Here's how the part is built. I have some questions about the finished solid (model axes, mm). Round coordinates to 2 decimals unless told otherwise and drop trailing zeros. Write each loop counter-clockwise with the first axis right and the second up, starting at its lowest first coordinate (ties: lowest second). Pieces come first, ordered by that corner, then holes. Notation, with made-up numbers: (-24, 23) - (6, 23) arc R26 ccw to (6, 48) - close; hole circle Ø8 at (8.5, 84.25). An arc over 180 degrees is marked (long way). One line per question, with ' | ' between items. Start each with the question number.
(1) Imagine slicing it at A-A (y = 79). Write out the boundary of the cut face in (x, z), plus the area to 3 significant figures.
(2) Thinking about a two-plate mould opening in Z: for faces 1 (the cylindrical face through (10.99, 81.2, -249.76)), 2 (the flat face through (3, 150, -3)), 3 (the flat face through (3, 25, -3)), which applies, pulls with the +Z half, pulls with the -Z half, needs draft (parallel to the pull), parting line crosses it, or undercut?
(3) Will these pins go through, and if not, where does the flat tip stop? pin 1 (12 mm diameter, centred on x = -47, y = 124.5, fed in from +Z); pin 2 (1.5 mm diameter, centred on x = -129.5, y = 117, fed in from -Z); pin 3 (6 mm diameter, centred on x = 148.5, z = 75.5, fed in from -Y).
(4) If I drill on L1, parallel to Y at x = -16, z = 130; L2, parallel to X at y = 20, z = 2; L3, parallel to X at y = 98, z = -17, over which ranges is the centre line in solid material (lowest first)?
(5) Imagine slicing it at B-B (y = 113.5). Write out the boundary of the cut face in (x, z), plus the area to 3 significant figures.
from build123d import *

# Parameters (mm, degrees)
SKETCH_4_R          = 250
EXTRUDE_2_DEPTH     = 150
FILLET_1_R          = 60
FILLET_2_R          = 47
SKETCH_16_R         = 190
CUT_EXTRUDE_1_DEPTH = 25
FILLET_3_R          = 25


with BuildPart() as part:
    # 草图4 → 凸台-拉伸2 (new body)
    with BuildSketch(Plane(origin=(0, 0, 0), x_dir=(1, 0, 0), z_dir=(0, 1, 0))):
        with Locations(Location((0, 0, 0), (0, 0, 270))):
            Circle(SKETCH_4_R)
    extrude(amount=EXTRUDE_2_DEPTH)

    # 圆角1
    fillet_1_edges = [part.edges().sort_by_distance(p)[0] for p in [
        (0, 0, -250),
    ]]
    fillet(fillet_1_edges, radius=FILLET_1_R)

    # 圆角2
    fillet_2_edges = [part.edges().sort_by_distance(p)[0] for p in [
        (0, 150, -250),
    ]]
    fillet(fillet_2_edges, radius=FILLET_2_R)

    # 草图16 → 切除-拉伸1 (cut)
    with BuildSketch(Plane(origin=(0, 0, 0), x_dir=(1, 0, 0), z_dir=(0, 1, 0))):
        with Locations(Location((0, 0, 0), (0, 0, 270))):
            Circle(SKETCH_16_R)
    extrude(amount=CUT_EXTRUDE_1_DEPTH, mode=Mode.SUBTRACT)

    # 圆角3
    # the kernel refuses this fillet: 25 mm, written as the material it takes off along each edge
    with BuildSketch(Plane(origin=(0, 0, 0), x_dir=(0, 0, 1), z_dir=(-1, 0, 0))) as fillet_3_piece_1:
        with BuildLine():
            CenterArc((213.35124434, 33.928571429), FILLET_3_R, 200.924832428, 110.924832428)
            Line((190, 25), (189.532975113, 24.821428571))
            ThreePointArc((189.532975113, 24.821428571), (189.5, 12.5), (189.5, 0))
            Line((189.5, 0), (190, -0.5))
            ThreePointArc((190, -0.5), (211.607142857, 3.489988696), (230.364293788, 14.933673469))
            Line((230.364293788, 14.933673469), (230.030704584, 15.306122449))
        make_face()
    revolve(axis=Axis((0, 0, 0), (0, 1, 0)), mode=Mode.SUBTRACT)

    # 倒角1
    # the kernel refuses this chamfer: 17.333818879, 10 mm, written as the material it adds along each edge
    with BuildSketch(Plane(origin=(0, 25, 0), x_dir=(0, 0, 1), z_dir=(-1, 0, 0))) as chamfer_1_piece_1:
        with BuildLine():
            Line((197.061199814, -10.000793021), (184.322097601, 0.439495442))
            Line((184.322097601, 0.439495442), (184.322097601, 0.786171819))
            ThreePointArc((184.322097601, 0.786171819), (187.161048801, 0.346676378), (190, 0.346676378))
            Line((190, 0.346676378), (190.323812992, 0.123812992))
            ThreePointArc((190.323812992, 0.123812992), (193.180553266, -5.246391965), (197.294531196, -9.744392989))
            Line((197.294531196, -9.744392989), (197.061199814, -10.000793021))
        make_face()
    revolve(axis=Axis((0, 25, 0), (0, 1, 0)))


solid = part.part
Check sheet entries:
1) outline: circle Ø500 at (0, 0) | area: 196,000 mm^2
2) face 1: parting line crosses it | face 2: needs draft | face 3: undercut
3) pin 1: z = 243.14 | pin 2: z = -211.88 | pin 3: y = 25
4) L1: 25 to 150 | L2: -234.71 to -190.95, 190.95 to 234.71 | L3: -249.42 to 249.42
5) outline: circle Ø497.62 at (0, 0) | area: 194,000 mm^2
